Geometry check sheet. Reference: the model listing, model coordinates, mm. Face numbers are marked on the shaded views. A direction names the side the tool comes from. Coordinates: 2 decimals unless noted, no trailing zeros. Order: outer loops, then holes, each group sorted by start corner. A loop starts at its lowest first (then second) coordinate and runs counter-clockwise, first axis right, second up. Notation, with made-up numbers: (-18, 11.25) - (-13, 11.25) arc R20 cw to (-13, 27.25) - close; hole circle Ø7 at (24, -6.5). An arc over 180 degrees is marked (long way). Return JSON: item names as keys, results as strings. Group by question number.
Item 1: Scan lines: probe 1 along Y at (x, z) = (0, 1.15); probe 2 along Y at (x, z) = (0, 55); probe 3 along Z at (x, y) = (2, 0). Record each from-to range of solid material in increasing order.
Item 2: Gauge pin test, flat ends, axial feed: pin 1 (4 mm diameter, centred on y = -6.5, z = 64, fed in from -X); pin 2 (4 mm diameter, centred on x = -4.5, z = 64, fed in from +Y); pin 3 (1.5 mm diameter, centred on x = 1, z = 50.5, fed in from +Y); pin 4 (2.5 mm diameter, centred on x = 0, y = 0, fed in from +Z). Record the tip position at first contact, or that the pin passes through.
Item 3: Section check C-C on z = 26. Enter the section's corners in (x, y).
Item 4: Section check A-A on y = 0. Enter the section's corners in (x, z), then the cut area to 3 significant figures.
Item 5: Tool access check on the marked faces 1 and 2. Record the directions out of +Z, -Z, +X, -X, +Y, -Y that give a thin tool (end or side, any length) a straight path to the whole face; none if there is none.
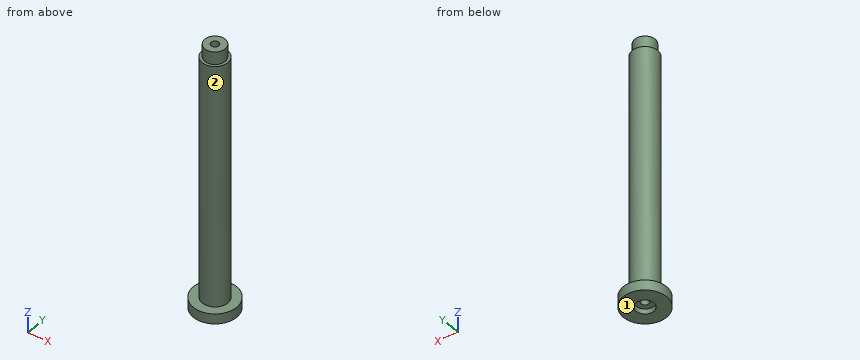
from build123d import *

# Parameters (mm, degrees)
F0_R     = 8.5
F1_DEPTH = 4
F2_R     = 5
F3_DEPTH = 100
F4_W     = 4
F4_H     = 5
F6_R     = 3.5
F7_DEPTH = 2
F8_R     = 1.5
F9_DEPTH = 118.6


with BuildPart() as f1:
    # F0 (on Top) → F1 (new body)
    with BuildSketch(Plane.XY):
        Circle(F0_R)
    extrude(amount=F1_DEPTH)

    # F2 (on Top) → F3 (join)
    with BuildSketch(Plane.XY):
        Circle(F2_R)
    extrude(amount=F3_DEPTH)

    # F4 (on Right) → F5 (revolve)
    with BuildSketch(Plane.YZ):
        with Locations((2, 102.5)):
            Rectangle(F4_W, F4_H)
    revolve(axis=Axis((0, 0, 102.5), (0, 0, -1)))

    # F6 (on face) → F7 (cut)
    with BuildSketch(Plane(origin=(0, 0, 0), x_dir=(1, 0, 0), z_dir=(0, 0, -1))):
        Circle(F6_R)
    extrude(amount=-F7_DEPTH, mode=Mode.SUBTRACT)

    # F8 (on face) → F9 (cut)
    with BuildSketch(Plane.XY.offset(105)):
        Circle(F8_R)
    extrude(amount=-F9_DEPTH, mode=Mode.SUBTRACT)


solid = f1.part
Computed:
{
 "1": {"probe 1": "y = -8.5 to -3.5, 3.5 to 8.5", "probe 2": "y = -5 to -1.5, 1.5 to 5", "probe 3": "z = 2 to 105"},
 "2": {"pin 1": "stops at x = -2.18", "pin 2": "stops at y = 4.33", "pin 3": "stops at y = 4.99", "pin 4": "passes through"},
 "3": {"outline": "circle Ø10 at (0, 0); hole circle Ø3 at (0, 0)"},
 "4": {"outline": "(-8.5, 0) - (-3.5, 0) - (-3.5, 2) - (-1.5, 2) - (-1.5, 105) - (-4, 105) - (-4, 100) - (-5, 100) - (-5, 4) - (-8.5, 4) - close; (1.5, 2) - (3.5, 2) - (3.5, 0) - (8.5, 0) - (8.5, 4) - (5, 4) - (5, 100) - (4, 100) - (4, 105) - (1.5, 105) - close", "area": "745 mm²"},
 "5": {"face 1": "-Z, +X, -X, +Y, -Y", "face 2": "+Z"}
}
